from build123d import *

# Parameters (mm, degrees)
SKETCH1_W           = 3.175
SKETCH1_H           = 25.4
BOSS_EXTRUDE1_DEPTH = 3.175


with BuildPart() as part:
    # Sketch1 → Boss-Extrude1 (new body)
    with BuildSketch(Plane.XY):
        Polygon((65.314285714, 135.64235), (65.214285714, 135.64235), (51.807142857, 135.64235), (51.707142857, 135.64235), (51.707142857, 138.81735), (39.007142857, 138.81735), (39.007142857, 135.64235), (38.907142857, 135.64235), (25.5, 135.64235), (25.4, 135.64235), (25.4, 138.81735), (12.7, 138.81735), (12.7, 135.64235), (12.6, 135.64235), (0, 135.64235), (0, 0), (12.6, 0), (12.7, 0), (12.7, -3.175), (25.4, -3.175), (25.4, 0), (25.5, 0), (38.907142857, 0), (39.007142857, 0), (39.007142857, -3.175), (51.707142857, -3.175), (51.707142857, 0), (51.807142857, 0), (65.214285714, 0), (65.314285714, 0), (65.314285714, -3.175), (78.014285714, -3.175), (78.014285714, 0), (78.114285714, 0), (91.521428571, 0), (91.621428571, 0), (91.621428571, -3.175), (104.321428571, -3.175), (104.321428571, 0), (104.421428571, 0), (117.828571429, 0), (117.928571429, 0), (117.928571429, -3.175), (130.628571429, -3.175), (130.628571429, 0), (130.728571429, 0), (144.135714286, 0), (144.235714286, 0), (144.235714286, -3.175), (156.935714286, -3.175), (156.935714286, 0), (157.035714286, 0), (170.442857143, 0), (170.542857143, 0), (170.542857143, -3.175), (183.242857143, -3.175), (183.242857143, 0), (183.342857143, 0), (196.75, 0), (196.85, 0), (196.85, -3.175), (209.55, -3.175), (209.55, 0), (209.65, 0), (223.057142857, 0), (223.157142857, 0), (223.157142857, -3.175), (235.857142857, -3.175), (235.857142857, 0), (235.957142857, 0), (249.364285714, 0), (249.464285714, 0), (249.464285714, -3.175), (262.164285714, -3.175), (262.164285714, 0), (262.264285714, 0), (275.671428571, 0), (275.771428571, 0), (275.771428571, -3.175), (288.471428571, -3.175), (288.471428571, 0), (288.571428571, 0), (301.978571429, 0), (302.078571429, 0), (302.078571429, -3.175), (314.778571429, -3.175), (314.778571429, 0), (314.878571429, 0), (328.285714286, 0), (328.385714286, 0), (328.385714286, -3.175), (341.085714286, -3.175), (341.085714286, 0), (341.185714286, 0), (354.592857143, 0), (354.692857143, 0), (354.692857143, -3.175), (367.392857143, -3.175), (367.392857143, 0), (367.492857143, 0), (380.9, 0), (381, 0), (381, -3.175), (393.7, -3.175), (393.7, 0), (393.8, 0), (406.4, 0), (406.4, 135.64235), (393.8, 135.64235), (393.7, 135.64235), (393.7, 138.81735), (381, 138.81735), (381, 135.64235), (380.9, 135.64235), (367.492857143, 135.64235), (367.392857143, 135.64235), (367.392857143, 138.81735), (354.692857143, 138.81735), (354.692857143, 135.64235), (354.592857143, 135.64235), (341.185714286, 135.64235), (341.085714286, 135.64235), (341.085714286, 138.81735), (328.385714286, 138.81735), (328.385714286, 135.64235), (328.285714286, 135.64235), (314.878571429, 135.64235), (314.778571429, 135.64235), (314.778571429, 138.81735), (302.078571429, 138.81735), (302.078571429, 135.64235), (301.978571429, 135.64235), (288.571428571, 135.64235), (288.471428571, 135.64235), (288.471428571, 138.81735), (275.771428571, 138.81735), (275.771428571, 135.64235), (275.671428571, 135.64235), (262.264285714, 135.64235), (262.164285714, 135.64235), (262.164285714, 138.81735), (249.464285714, 138.81735), (249.464285714, 135.64235), (249.364285714, 135.64235), (235.957142857, 135.64235), (235.857142857, 135.64235), (235.857142857, 138.81735), (223.157142857, 138.81735), (223.157142857, 135.64235), (223.057142857, 135.64235), (209.65, 135.64235), (209.55, 135.64235), (209.55, 138.81735), (196.85, 138.81735), (196.85, 135.64235), (196.75, 135.64235), (183.342857143, 135.64235), (183.242857143, 135.64235), (183.242857143, 138.81735), (170.542857143, 138.81735), (170.542857143, 135.64235), (170.442857143, 135.64235), (157.035714286, 135.64235), (156.935714286, 135.64235), (156.935714286, 138.81735), (144.235714286, 138.81735), (144.235714286, 135.64235), (144.135714286, 135.64235), (130.728571429, 135.64235), (130.628571429, 135.64235), (130.628571429, 138.81735), (117.928571429, 138.81735), (117.928571429, 135.64235), (117.828571429, 135.64235), (104.421428571, 135.64235), (104.321428571, 135.64235), (104.321428571, 138.81735), (91.621428571, 138.81735), (91.621428571, 135.64235), (91.521428571, 135.64235), (78.114285714, 135.64235), (78.014285714, 135.64235), (78.014285714, 138.81735), (65.314285714, 138.81735), align=None)
        with Locations((401.6375, 93.221175)):
            Rectangle(SKETCH1_W, SKETCH1_H, mode=Mode.SUBTRACT)
        with Locations((401.6375, 42.421175)):
            Rectangle(SKETCH1_W, SKETCH1_H, mode=Mode.SUBTRACT)
        with Locations((4.7625, 93.221175)):
            Rectangle(SKETCH1_W, SKETCH1_H, mode=Mode.SUBTRACT)
        with Locations((4.7625, 42.421175)):
            Rectangle(SKETCH1_W, SKETCH1_H, mode=Mode.SUBTRACT)
    extrude(amount=BOSS_EXTRUDE1_DEPTH)


solid = part.part
Here's how the part is built. I have some questions about the finished solid (model axes, mm). Coordinates: 2 decimals unless noted, no trailing zeros. Loops run counter-clockwise (first coordinate to the right, second up) from the corner with the lowest first, then second, coordinate; pieces in that order, holes last. Notation, with made-up numbers: (49.5, 67.25) -> (93.5, 67.25) arc R15 cw to (93.5, 74.25) -> close; hole circle Ø3 at (-10, 82.25). An arc over 180 degrees is marked (long way). Use one line per item in the form item = value. Start each with the question number.
(1) If we section it at C-C (z = 1.55): Give the number of separate pieces and of enclosed holes in the cut face, then the cut area to 3 significant figures.
(2) Please list where these lines run through material, in increasing order: line 1 along X through (y, z) = (84.5, 2.9) (3 decimals); line 2 along Y through (x, z) = (321.5, 1.9).
(3) If we section it at B-B (x = 241): Please give me the cut outline in (y, z) (3 decimals), then the cut area to 3 significant figures.
(4) If we section it at A-A (y = 89): Please give me the cut outline in (x, z) (3 decimals).
(5) Will these pins go through, and if not, where does the flat tip stop? pin 1 (1.6 mm diameter, centred on x = 4, z = 2, fed in from +Y); pin 2 (1 mm diameter, centred on x = 83.5, z = 2, fed in from -Y); pin 3 (1 mm diameter, centred on y = -2, z = 1.5, fed in from +X).
Verdict:
q1.separate_pieces = 1
q1.enclosed_holes = 4
q1.area = 56,000 mm²
q2.line_1 = 0 to 3.175, 6.35 to 400.05, 403.225 to 406.4
q2.line_2 = 0 to 135.64
q3.outline = (0, 0) -> (135.642, 0) -> (135.642, 3.175) -> (0, 3.175) -> close
q3.area = 431 mm²
q4.outline = (0, 0) -> (3.175, 0) -> (3.175, 3.175) -> (0, 3.175) -> close; (6.35, 0) -> (400.05, 0) -> (400.05, 3.175) -> (6.35, 3.175) -> close; (403.225, 0) -> (406.4, 0) -> (406.4, 3.175) -> (403.225, 3.175) -> close
q5.pin_1 = 135.64
q5.pin_2 = 0
q5.pin_3 = 393.7
